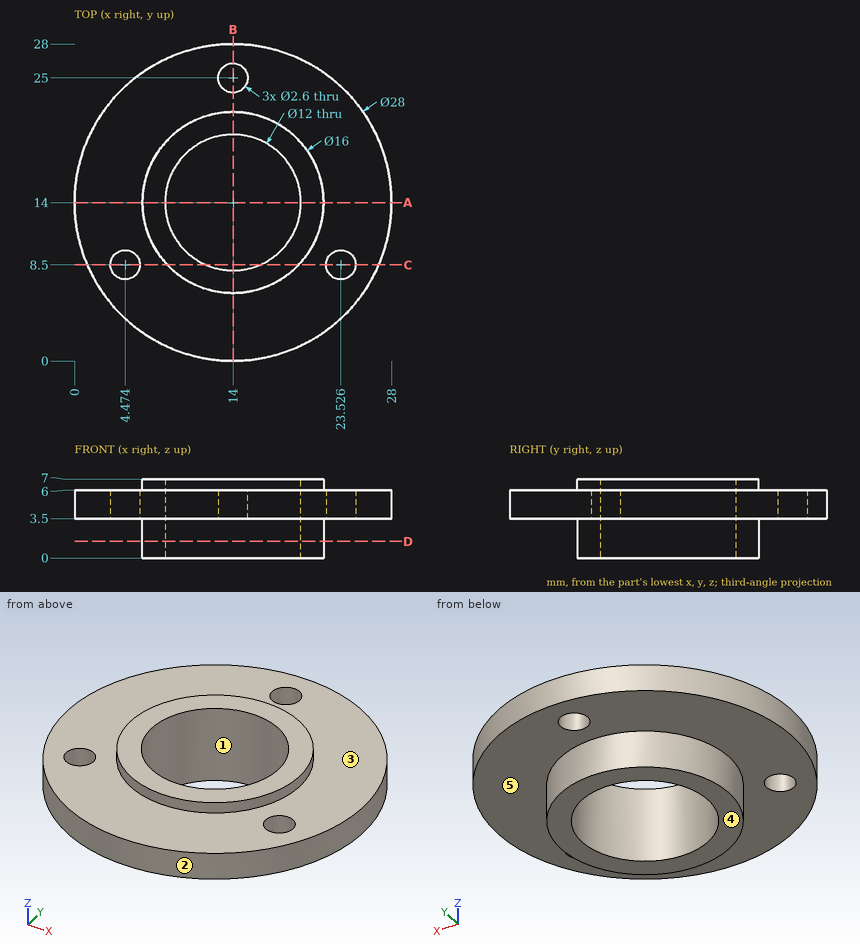
Source: three-view drawing plus pictorial views. Frame: mm from the lowest corner of the part. A direction names the side the tool comes from. Round coordinates to 2 decimals unless told otherwise and drop trailing zeros. Order: outer loops, then holes, each group sorted by start corner. A loop starts at its lowest first (then second) coordinate and runs counter-clockwise, first axis right, second up. Notation, with made-up numbers: (63.25, 34) - (106.25, 34) arc R21 ccw to (106.25, 47) - close; hole circle Ø6 at (7.25, 8). An arc over 180 degrees is marked (long way). Answer in a Markdown table with one row per item.
Item 1: Section query C-C (y = 8.5). Return the cut outline in (x, z).
Model answer:
| item | result |
|---|---|
| outline | (1.13, 3.5) - (3.17, 3.5) - (3.17, 6) - (1.13, 6) - close; (5.77, 3.5) - (8.19, 3.5) - (8.19, 0) - (11.6, 0) - (11.6, 7) - (8.19, 7) - (8.19, 6) - (5.77, 6) - close; (16.4, 0) - (19.81, 0) - (19.81, 3.5) - (22.23, 3.5) - (22.23, 6) - (19.81, 6) - (19.81, 7) - (16.4, 7) - close; (24.83, 3.5) - (26.87, 3.5) - (26.87, 6) - (24.83, 6) - close |
Item 2: Section query B-B (x = 14). Return the cut outline in (y, z), then the cut area to 3 significant figures.
Model answer:
| item | result |
|---|---|
| outline | (0, 3.5) - (6, 3.5) - (6, 0) - (8, 0) - (8, 7) - (6, 7) - (6, 6) - (0, 6) - close; (20, 0) - (22, 0) - (22, 3.5) - (23.7, 3.5) - (23.7, 6) - (22, 6) - (22, 7) - (20, 7) - close; (26.3, 3.5) - (28, 3.5) - (28, 6) - (26.3, 6) - close |
| area | 51.5 mm² |
Item 3: Pin query (flat end, axial travel): pin 1 (2.5 mm diameter, centred on x = 23.53, y = 8.5, fed in from +Z); pin 2 (2 mm diameter, centred on y = 20, z = 5.5, fed in from +X); pin 3 (3 mm diameter, centred on x = 8, z = 3, fed in from +Y); pin 4 (2 mm diameter, centred on y = 20.5, z = 3.5, fed in from -X) (1 decimal). Return the tip coordinate at first contact, or that it passes through.
Model answer:
| item | result |
|---|---|
| pin 1 | passes through |
| pin 2 | stops at x = 27.08 |
| pin 3 | stops at y = 27.23 |
| pin 4 | stops at x = 1.1 |
Item 4: Line query: line 1 (Y direction, x = 14, z = 4.5); line 2 (Y direction, x = 13, z = 4.5) (1 decimal); line 3 (Z direction, x = 25.5, y = 19.5). Output: solid intervals per line, ascending.
Model answer:
| item | result |
|---|---|
| line 1 | y = 0 to 8, 20 to 23.7, 26.3 to 28 |
| line 2 | y = 0 to 8.1, 19.9 to 24.2, 25.8 to 28 |
| line 3 | z = 3.5 to 6 |
Item 5: Section query D-D (z = 1.5). Return the cut outline in (x, y).
Model answer:
| item | result |
|---|---|
| outline | circle Ø16 at (14, 14); hole circle Ø12 at (14, 14) |
Item 6: Reachability of the marked faces 4 and 5 from +Z, -Z, +X, -X, +Y, -Y: full face, straight path, thin tool, end or side. Return the list, or none.
Model answer:
| item | result |
|---|---|
| face 4 | -Z, +X, -X, +Y, -Y |
| face 5 | -Z |
Item 7: Section query A-A (y = 14). Return the cut outline in (x, z), then the cut area to 3 significant figures.
Model answer:
| item | result |
|---|---|
| outline | (0, 3.5) - (6, 3.5) - (6, 0) - (8, 0) - (8, 7) - (6, 7) - (6, 6) - (0, 6) - close; (20, 0) - (22, 0) - (22, 3.5) - (28, 3.5) - (28, 6) - (22, 6) - (22, 7) - (20, 7) - close |
| area | 58.0 mm² |
Item 8: Mould query, pull axis Y, two halves, no side actions, for the marked faces 1, 2 and 3. Classes: released by +Y, released by -Y, zero draft, split by the parting line, or undercut.
Model answer:
| item | result |
|---|---|
| face 1 | undercut |
| face 2 | split by the parting line |
| face 3 | zero draft |
